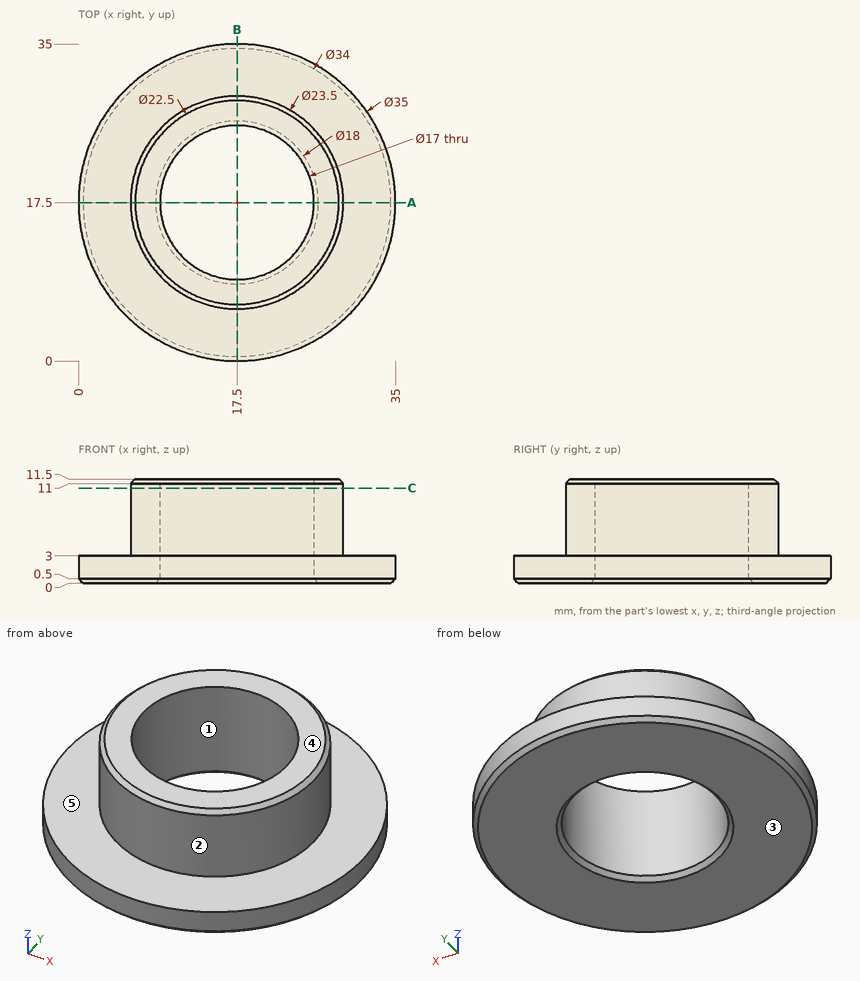
Verification items for this drawing (mm, ordinates from the low corner). A direction names the side the tool comes from. Coordinates: 2 decimals unless noted, no trailing zeros. Write each loop counter-clockwise with the first axis right and the second up, starting at its lowest first coordinate (ties: lowest second). Pieces come first, ordered by that corner, then holes. Notation, with made-up numbers: M 44,78 L 64,78 A21 cw 64,115 Z; hole C 48,-1.5 d5. An arc over 180 degrees is marked long. Use one line per item in the form item = value. Start each with the question number.
1) Section check A-A on y = 17.5. Enter the section's corners in (x, z).
2) Thickness scan on probe 1 along Y at (x, z) = (17.5, 7); probe 2 along Z at (x, y) = (31, 12.5); probe 3 along Y at (x, z) = (12, 6.25). Record the ranges inside material, lowest first. Write a range as from..to.
3) Section check C-C on z = 10.5. Enter the section's corners in (x, y), and give its area (3 significant figures).
4) Release check for a two-part mould opening along Y. For the marked faces 1, 2 and 3 record: pulls with the +Y half, pulls with the -Y half, needs draft (parallel to the pull), parting line crosses it, or undercut.
5) Go/stop test with flat-tipped pins: pin 1 Ø2 at (x, z) = (31.5, 3) entering from -Y; pin 2 Ø3 at (x, z) = (28.5, 5) entering from +Y. Record where each tip stops, or that it passes through.
6) Set-up check for the marked faces 4 and 5: record each of +Z, -Z, +X, -X, +Y, -Y from which the full face is reachable in a straight line by a thin tool's end or side.
Responses:
q1.outline = M 0,0.5 L 0.5,0 L 8.5,0 L 9,0.5 L 9,11.5 L 6.25,11.5 L 5.75,11 L 5.75,3 L 0,3 Z; M 26,0.5 L 26.5,0 L 34.5,0 L 35,0.5 L 35,3 L 29.25,3 L 29.25,11 L 28.75,11.5 L 26,11.5 Z
q2.probe_1 = 5.75..9, 26..29.25
q2.probe_2 = 0..3
q2.probe_3 = 7.12..11.02, 23.98..27.88
q3.outline = C 17.5,17.5 d23.5; hole C 17.5,17.5 d17
q3.area = 207 mm2
q4.face_1 = undercut
q4.face_2 = parting line crosses it
q4.face_3 = needs draft
q5.pin_1 = 5.78
q5.pin_2 = 24.41
q6.face_4 = +Z, +X, -X, +Y, -Y
q6.face_5 = +Z
